Design review of the part built by this model. Coordinates are the model's own, in mm. Face numbers are marked on the shaded views. A direction names the side the tool comes from. Coordinates: 2 decimals unless noted, no trailing zeros. Loops run counter-clockwise (first coordinate to the right, second up) from the corner with the lowest first, then second, coordinate; pieces in that order, holes last. Notation, with made-up numbers: (17.5, 31) - (42.5, 31) arc R20 cw to (42.5, 69) - close; hole circle Ø2 at (74.25, 4). An arc over 180 degrees is marked (long way). One line per question, with ' | ' between items.
from build123d import *

# Parameters (mm, degrees)
F1_DEPTH = 3.175
F3_DEPTH = 12.7
F5_DEPTH = 12.7
F6_R     = 10.795
F7_DEPTH = 12.7


with BuildPart() as f1:
    # F0 (on Top) → F1 (new body)
    with BuildSketch(Plane.XY):
        with BuildLine():
            Line((72.204018, 53.623151), (86.545982, 79.726849))
            ThreePointArc((86.545982, 79.726849), (86.245899, 98.599329), (69.85, 107.95))
            Line((69.85, 107.95), (38.1, 107.95))
            Line((38.1, 107.95), (38.1, 95.25))
            Line((38.1, 95.25), (-38.1, 95.25))
            Line((-38.1, 95.25), (-38.1, 107.95))
            Line((-38.1, 107.95), (-69.85, 107.95))
            ThreePointArc((-69.85, 107.95), (-86.245899, 98.599329), (-86.545982, 79.726849))
            Line((-86.545982, 79.726849), (-72.204018, 53.623151))
            ThreePointArc((-72.204018, 53.623151), (-72.504101, 34.750671), (-88.9, 25.4))
            Line((-88.9, 25.4), (-103.66375, 25.4))
            Line((-103.66375, 25.4), (-107.95, 6.35))
            Line((-107.95, 6.35), (-107.95, -6.35))
            Line((-107.95, -6.35), (-102.467009, -25.4))
            Line((-102.467009, -25.4), (-82.55, -25.4))
            ThreePointArc((-82.55, -25.4), (-70.758346, -33.383338), (-73.791379, -47.296552))
            Line((-73.791379, -47.296552), (-82.987931, -56.055172))
            ThreePointArc((-82.987931, -56.055172), (-87.537481, -76.924992), (-69.85, -88.9))
            Line((-69.85, -88.9), (-41.275, -88.9))
            Line((-41.275, -88.9), (-41.275, -95.25))
            Line((-41.275, -95.25), (41.275, -95.25))
            Line((41.275, -95.25), (41.275, -88.9))
            Line((41.275, -88.9), (69.85, -88.9))
            ThreePointArc((69.85, -88.9), (87.537481, -76.924992), (82.987931, -56.055172))
            Line((82.987931, -56.055172), (73.791379, -47.296552))
            ThreePointArc((73.791379, -47.296552), (70.758346, -33.383338), (82.55, -25.4))
            Line((82.55, -25.4), (102.467009, -25.4))
            Line((102.467009, -25.4), (107.95, -6.35))
            Line((107.95, -6.35), (107.95, 6.35))
            Line((107.95, 6.35), (103.66375, 25.4))
            Line((103.66375, 25.4), (88.9, 25.4))
            ThreePointArc((88.9, 25.4), (72.504101, 34.750671), (72.204018, 53.623151))
        make_face()
    extrude(amount=F1_DEPTH)

    # F2 (on face) → F3 (join)
    with BuildSketch(Plane.XY.offset(3.175)):
        with BuildLine():
            Line((-38.1, 82.55), (-54.266603, 82.55))
            ThreePointArc((-54.266603, 82.55), (-81.748839, 100.798839), (-63.5, 73.316603))
            Line((-63.5, 73.316603), (-63.5, 25.4))
            Line((-63.5, 25.4), (-88.9, 25.4))
            Line((-88.9, 25.4), (-95.25, 25.4))
            ThreePointArc((-95.25, 25.4), (-99.740128, 23.540128), (-101.6, 19.05))
            Line((-101.6, 19.05), (-101.6, -19.05))
            ThreePointArc((-101.6, -19.05), (-99.740128, -23.540128), (-95.25, -25.4))
            Line((-95.25, -25.4), (-82.55, -25.4))
            Line((-82.55, -25.4), (-63.5, -25.4))
            Line((-63.5, -25.4), (-63.5, -54.266603))
            ThreePointArc((-63.5, -54.266603), (-86.450842, -72.602597), (-58.81031, -82.55))
            Line((-58.81031, -82.55), (-38.1, -82.55))
            Line((-38.1, -82.55), (-38.1, -95.25))
            Line((-38.1, -95.25), (38.1, -95.25))
            Line((38.1, -95.25), (38.1, -82.55))
            Line((38.1, -82.55), (58.81031, -82.55))
            ThreePointArc((58.81031, -82.55), (86.450842, -72.602597), (63.5, -54.266603))
            Line((63.5, -54.266603), (63.5, -25.4))
            Line((63.5, -25.4), (82.55, -25.4))
            Line((82.55, -25.4), (95.25, -25.4))
            ThreePointArc((95.25, -25.4), (99.740128, -23.540128), (101.6, -19.05))
            Line((101.6, -19.05), (101.6, 19.05))
            ThreePointArc((101.6, 19.05), (99.740128, 23.540128), (95.25, 25.4))
            Line((95.25, 25.4), (88.9, 25.4))
            Line((88.9, 25.4), (63.5, 25.4))
            Line((63.5, 25.4), (63.5, 73.316603))
            ThreePointArc((63.5, 73.316603), (81.748839, 100.798839), (54.266603, 82.55))
            Line((54.266603, 82.55), (38.1, 82.55))
            Line((38.1, 82.55), (38.1, 95.25))
            Line((38.1, 95.25), (-38.1, 95.25))
            Line((-38.1, 95.25), (-38.1, 82.55))
        make_face()
    extrude(amount=F3_DEPTH)

    # F4 (on face) → F5 (cut)
    with BuildSketch(Plane.XY.offset(15.875)):
        Polygon((-35.179, 76.2), (-57.15, 76.2), (-57.15, 19.05), (-91.44, 19.05), (-91.44, -19.05), (-57.15, -19.05), (-57.15, -76.2), (-35.179, -76.2), (-35.179, -92.075), (35.179, -92.075), (35.179, -76.2), (57.15, -76.2), (57.15, -19.05), (91.44, -19.05), (91.44, 19.05), (57.15, 19.05), (57.15, 76.2), (35.179, 76.2), (35.179, 92.075), (-35.179, 92.075), align=None)
    extrude(amount=-F5_DEPTH, mode=Mode.SUBTRACT)

    # F6 (on face) → F7 (cut)
    with BuildSketch(Plane.XY.offset(15.875)):
        with Locations((-69.85, -69.85)):
            Circle(F6_R)
        with Locations((-69.85, 88.9)):
            Circle(F6_R)
        with Locations((69.85, 88.9)):
            Circle(F6_R)
        with Locations((69.85, -69.85)):
            Circle(F6_R)
    extrude(amount=-F7_DEPTH, mode=Mode.SUBTRACT)


solid = f1.part
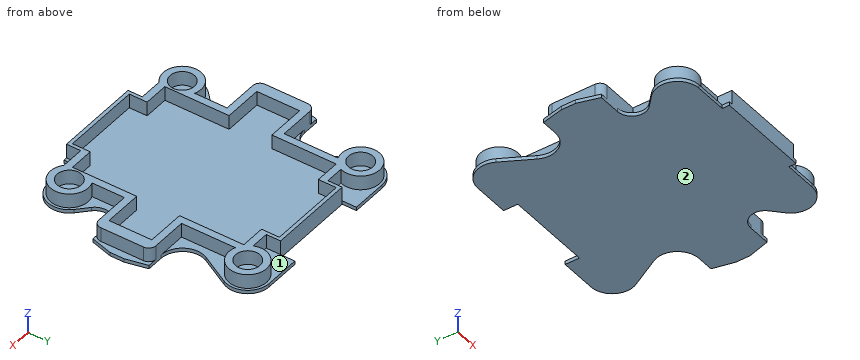
Q1. For pin 1 (3.5 mm diameter, centred on x = 54, z = 2, fed in from -Y); pin 2 (1 mm diameter, centred on y = -93.5, z = 1, fed in from +X) (3 decimals); pin 3 (5 mm diameter, centred on x = -83.5, z = 9.5, fed in from +Y), all flat-tipped, find the tip position at first contact; note any pin that passes through.
Returned:
pin 1: stops at y = -88.9 | pin 2: stops at x = 41.275 | pin 3: stops at y = 101.5
Q2. Take a section at B-B (x = -4.5). Give the boundary of the cut face in (y, z) (3 decimals).
Returned:
outline: (-95.25, 0) - (95.25, 0) - (95.25, 15.875) - (92.075, 15.875) - (92.075, 3.175) - (-92.075, 3.175) - (-92.075, 15.875) - (-95.25, 15.875) - close
Q3. Take a section at D-D (y = 88.9). Give the boundary of the cut face in (x, z) (1 decimal).
Returned:
outline: (-88.9, 0) - (88.9, 0) - (88.9, 3.2) - (86.7, 3.2) - (86.7, 15.9) - (80.6, 15.9) - (80.6, 3.2) - (59.1, 3.2) - (59.1, 15.9) - (53, 15.9) - (53, 3.2) - (38.1, 3.2) - (38.1, 15.9) - (35.2, 15.9) - (35.2, 3.2) - (-35.2, 3.2) - (-35.2, 15.9) - (-38.1, 15.9) - (-38.1, 3.2) - (-53, 3.2) - (-53, 15.9) - (-59.1, 15.9) - (-59.1, 3.2) - (-80.6, 3.2) - (-80.6, 15.9) - (-86.7, 15.9) - (-86.7, 3.2) - (-88.9, 3.2) - close
Q4. To check wall thickness, follow line 1 along X through (y, z) = (-70, 7); line 2 along Y through (x, z) = (70.5, 12.25); line 3 along Y through (x, z) = (33.5, 8.25) (3 decimals). State the ranges of each line that lie inside material, in increasing order.
Returned:
line 1: x = -86.68 to -80.64, -59.06 to -57.15, 57.15 to 59.06, 80.64 to 86.68 | line 2: y = -86.66 to -80.63, -59.07 to -53.04, -25.4 to -19.05, 19.05 to 25.4, 72.09 to 78.12, 99.68 to 105.71 | line 3: y = -95.25 to -92.075, 92.075 to 95.25
Q5. Tool access review of the marked faces 1 and 2: name each direction out of +Z, -Z, +X, -X, +Y, -Y from which nothing blocks a thin tool from reaching the whole face with its end or side.
Returned:
face 1: +Z | face 2: -Z, +X, -X, +Y, -Y
Q6. Take a section at C-C (z = 8). State how many separate pieces and enclosed holes the cut face has, plus the area to 3 significant figures.
Returned:
separate pieces: 1 | enclosed holes: 5 | area: 6,000 mm²
